```python
from build123d import *

# Parameters (mm, degrees)
ESQUISSE1_W          = 36
ESQUISSE1_H          = 56
ESQUISSE1_R          = 1.6
BOARD_DEPTH          = 1.6
ESQUISSE2_W          = 8
ESQUISSE2_H          = 8
RS232_DEPTH          = 6
ESQUISSE3_W          = 5
ESQUISSE3_H          = 6
LIMIT_SWITCH_DEPTH   = 8
ESQUISSE4_W          = 18
ESQUISSE4_H          = 35.5
TEENSY_4_0_DEPTH     = 12
ESQUISSE5_W          = 9
ESQUISSE5_H          = 12
F_5V_REGULATOR_DEPTH = 10.4


with BuildPart() as part:
    # Esquisse1 → Board (new body)
    with BuildSketch(Plane.XY):
        with Locations((-18, 28)):
            Rectangle(ESQUISSE1_W, ESQUISSE1_H)
        with Locations((-31.5, 51.5)):
            Circle(ESQUISSE1_R, mode=Mode.SUBTRACT)
        with Locations((-4.5, 51.5)):
            Circle(ESQUISSE1_R, mode=Mode.SUBTRACT)
    extrude(amount=BOARD_DEPTH)

    # Esquisse2 → RS232 (add)
    with BuildSketch(Plane.XY.offset(1.6)):
        with Locations((-14, 52)):
            Rectangle(ESQUISSE2_W, ESQUISSE2_H)
    extrude(amount=RS232_DEPTH)

    # Esquisse3 → Limit switch (add)
    with BuildSketch(Plane.XY.offset(1.6)):
        with Locations((-2.5, 40.5)):
            Rectangle(ESQUISSE3_W, ESQUISSE3_H)
    extrude(amount=LIMIT_SWITCH_DEPTH)

    # Esquisse4 → Teensy 4.0 (add)
    with BuildSketch(Plane.XY.offset(1.6)):
        with Locations((-10.5, 19.25)):
            Rectangle(ESQUISSE4_W, ESQUISSE4_H)
    extrude(amount=TEENSY_4_0_DEPTH)

    # Esquisse5 → 5v regulator (add)
    with BuildSketch(Plane.XY.offset(1.6)):
        with Locations((-31.5, 31)):
            Rectangle(ESQUISSE5_W, ESQUISSE5_H)
    extrude(amount=F_5V_REGULATOR_DEPTH)


solid = part.part
```
Design review of the part built by this model. Coordinates are the model's own, in mm. A direction names the side the tool comes from. Round coordinates to 2 decimals unless told otherwise and drop trailing zeros. Order: outer loops, then holes, each group sorted by start corner. A loop starts at its lowest first (then second) coordinate and runs counter-clockwise, first axis right, second up. Notation, with made-up numbers: M 5.5,18 L 47.5,18 A34 ccw 47.5,57 Z; hole C 0,34 d10. An arc over 180 degrees is marked long. Put each result on its own line as item: value.
Q1. To check wall thickness, follow line 1 (Y direction, x = -11.5, z = 3); line 2 (Y direction, x = -31.5, z = 0.6); line 3 (X direction, y = 33.5, z = 7.5). State the ranges of each line that lie inside material, in increasing order.
Reported:
line 1: 1.5 to 37, 48 to 56
line 2: 0 to 49.9, 53.1 to 56
line 3: -36 to -27, -19.5 to -1.5
Q2. Consider section A-A (y = 51.5). State the section outline as (x, z) points.
Reported:
outline: M -36,0 L -33.1,0 L -33.1,1.6 L -36,1.6 Z; M -29.9,0 L -6.1,0 L -6.1,1.6 L -10,1.6 L -10,7.6 L -18,7.6 L -18,1.6 L -29.9,1.6 Z; M -2.9,0 L 0,0 L 0,1.6 L -2.9,1.6 Z
Q3. Consider section B-B (x = -31.5). State the section outline as (y, z) points.
Reported:
outline: M 0,0 L 49.9,0 L 49.9,1.6 L 37,1.6 L 37,12 L 25,12 L 25,1.6 L 0,1.6 Z; M 53.1,0 L 56,0 L 56,1.6 L 53.1,1.6 Z
Q4. Consider section C-C (y = 33). State the section outline as (x, z) points.
Reported:
outline: M -36,0 L 0,0 L 0,1.6 L -1.5,1.6 L -1.5,13.6 L -19.5,13.6 L -19.5,1.6 L -27,1.6 L -27,12 L -36,12 Z
Q5. Machinability: for faces 1 (the face through (-1.5, 19, 8)), 2 (the face through (-32, 25, 7)), 3 (the face through (-3, 37.5, 6)), 4 (the face through (-14, 52, 7.6)), 5 (the face through (-32, 31, 12)), which of the approach directions +Z, -Z, +X, -X, +Y, -Y give a long, thin tool a straight path to every point of the face, cutting with its end or side? Answer none if there is none.
Reported:
face 1: +Z, +X, -Y
face 2: +Z, -X, -Y
face 3: +Z, +X, -X
face 4: +Z, +X, -X, +Y
face 5: +Z, -X, +Y, -Y
Q6. Consider section D-D (x = -8.5). State the section outline as (y, z) points.
Reported:
outline: M 0,0 L 56,0 L 56,1.6 L 37,1.6 L 37,13.6 L 1.5,13.6 L 1.5,1.6 L 0,1.6 Z
Q7. Insertion check: pin 1 Ø4 at (x, z) = (-4.5, 11.5) entering from +Y; pin 2 Ø1.9 at (x, y) = (-4.5, 51.5) entering from +Z; pin 3 Ø6 at (x, y) = (-24.5, 22) entering from +Z; pin 4 Ø1.5 at (y, z) = (22, 5.5) entering from -X. Each pin has a flat end and moves straight along its axis. Give the tip position at first contact, or say it passes through.
Reported:
pin 1: y = 43.5
pin 2: through
pin 3: z = 1.6
pin 4: x = -19.5
